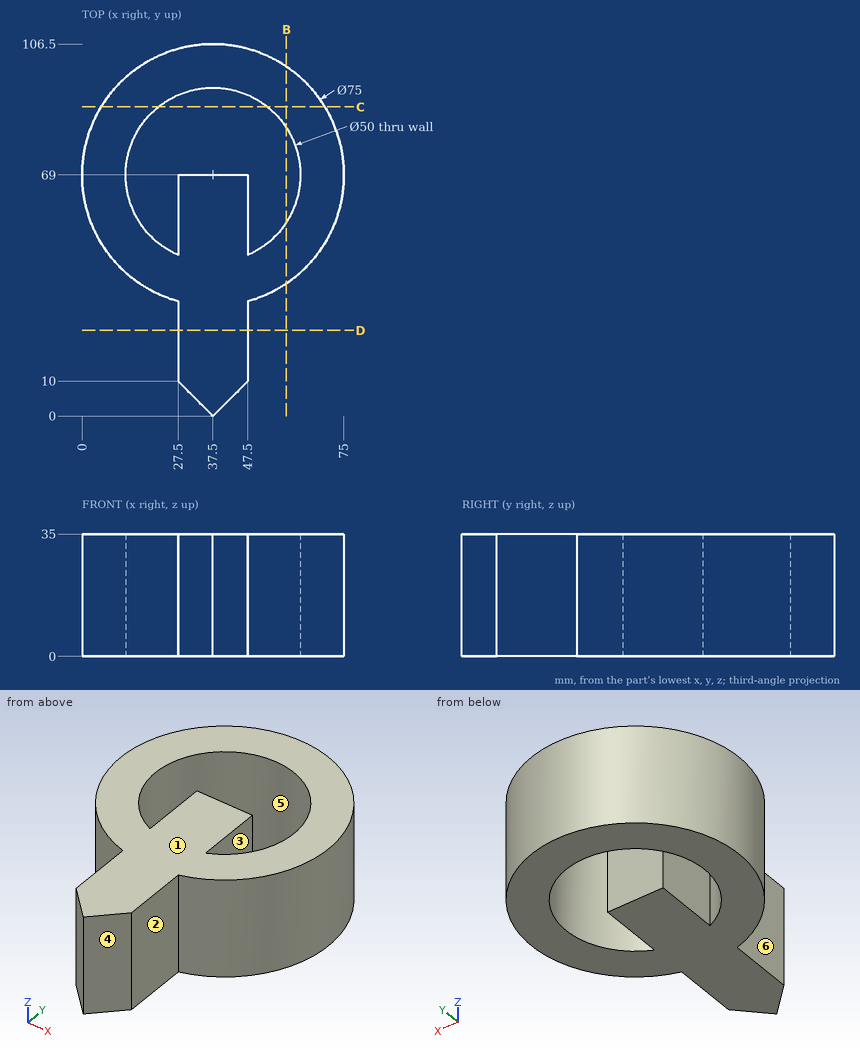
Source: three-view drawing plus pictorial views. Frame: mm from the lowest corner of the part. A direction names the side the tool comes from. Coordinates: 2 decimals unless noted, no trailing zeros. Order: outer loops, then holes, each group sorted by start corner. A loop starts at its lowest first (then second) coordinate and runs counter-clockwise, first axis right, second up. Notation, with made-up numbers: M 79.25,-4 L 133.25,-4 A23 ccw 133.25,29 Z; hole C 37,6.25 d3. An arc over 180 degrees is marked long. One line per question, with ' | ' between items. Start each with the question number.
Item 1: Cut plane D-D, the plane y = 24.5. Return the cut outline in (x, z).
Item 2: Set-up query: the marked faces 1, 2 and 3. Return all of +Z, -Z, +X, -X, +Y, -Y with unobstructed straight access to the full face (end or side cutting, diameter ignored); none if empty.
Item 3: Draft query along Y for the marked faces 4, 5 and 6. Return one class per face: released by +Y, released by -Y, zero draft, split by the parting line, or undercut.
Item 4: Pin query (flat end, axial travel): pin 1 Ø18.5 at (y, z) = (25.5, 17) entering from +X; pin 2 Ø10 at (x, z) = (17.5, 24) entering from +Y; pin 3 Ø4 at (x, z) = (9.5, 14.5) entering from +Y. Return the tip coordinate at first contact, or that it passes through.
Item 5: Ray query, probe 1 along X at (y, z) = (65, 15); probe 2 along X at (y, z) = (19, 33.5); probe 3 along X at (y, z) = (78, 7.5). Return the intervals inside material, ascending. Write a range as [from, to].
Item 6: Cut plane C-C, the plane y = 88.5. Return the cut outline in (x, z).
Item 7: Cut plane B-B, the plane x = 58.5. Return the cut outline in (y, z).
A:
1) outline: M 27.5,0 L 47.5,0 L 47.5,35 L 27.5,35 Z
2) face 1: +Z, +X, -X, +Y, -Y | face 2: +Z, -Z, +X, -Y | face 3: +Z, -Z
3) face 4: released by -Y | face 5: undercut | face 6: zero draft
4) pin 1: stops at x = 52.77 | pin 2: stops at y = 103.37 | pin 3: stops at y = 96.02
5) probe 1: x = [0.21, 12.82], [27.5, 47.5], [62.18, 74.79] | probe 2: x = [27.5, 47.5] | probe 3: x = [1.1, 14.18], [60.82, 73.9]
6) outline: M 5.47,0 L 21.86,0 L 21.86,35 L 5.47,35 Z; M 53.14,0 L 69.53,0 L 69.53,35 L 53.14,35 Z
7) outline: M 37.93,0 L 55.44,0 L 55.44,35 L 37.93,35 Z; M 82.56,0 L 100.07,0 L 100.07,35 L 82.56,35 Z
